Verification items for the finished model (mm, model axes). A direction names the side the tool comes from. Give positions to 0.01 mm unless a question says otherwise; leave off trailing zeros. Order: outer loops, then holes, each group sorted by start corner. A loop starts at its lowest first (then second) coordinate and runs counter-clockwise, first axis right, second up. Notation, with made-up numbers: M 65,19 L 116,19 A33 ccw 116,56 Z; hole C 72,47.5 d3. An arc over 180 degrees is marked long. Answer as a JSON object with one key per item and string values.
```python
from build123d import *

# Parameters (mm, degrees)
F0_W      = 65
F0_H      = 36
F1_DEPTH  = 23
F2_W      = 56
F2_H      = 26
F3_DEPTH  = 20
F4_R      = 2
F5_DEPTH  = 2
F6_R      = 1.25
F7_DEPTH  = 3
F8_R      = 1.25
F9_DEPTH  = 3
F10_R     = 6
F10_R_2   = 1.5
F11_DEPTH = 5
F12_W     = 24
F12_H     = 6
F13_DEPTH = 100


with BuildPart() as f1:
    # F0 (on Top) → F1 (new body)
    with BuildSketch(Plane.XY):
        Rectangle(F0_W, F0_H)
    extrude(amount=F1_DEPTH)

    # F2 (on face) → F3 (cut)
    with BuildSketch(Plane.XY.offset(23)):
        Rectangle(F2_W, F2_H)
    extrude(amount=-F3_DEPTH, mode=Mode.SUBTRACT)

    # F4 (on face) → F5 (join)
    with BuildSketch(Plane.XY.offset(3)):
        with Locations((-17, 9.5)):
            Circle(F4_R)
        with Locations((16.5, -9.5)):
            Circle(F4_R)
    extrude(amount=F5_DEPTH)

    # F6 (on face) → F7 (cut)
    with BuildSketch(Plane.XY.offset(5)):
        with Locations((-17, 9.5)):
            Circle(F6_R)
    extrude(amount=-F7_DEPTH, mode=Mode.SUBTRACT)

    # F8 (on face) → F9 (cut)
    with BuildSketch(Plane.XY.offset(5)):
        with Locations((16.5, -9.5)):
            Circle(F8_R)
    extrude(amount=-F9_DEPTH, mode=Mode.SUBTRACT)

    # F10 (on face) → F11 (join)
    with BuildSketch(Plane(origin=(0, 0, 0), x_dir=(1, 0, 0), z_dir=(0, 0, -1))):
        with Locations((-32.5, 18)):
            Circle(F10_R)
        with Locations((-34.5, 20)):
            Circle(F10_R_2, mode=Mode.SUBTRACT)
        with Locations((32.5, 18)):
            Circle(F10_R)
        with Locations((34.5, 20)):
            Circle(F10_R_2, mode=Mode.SUBTRACT)
        with Locations((32.5, -18)):
            Circle(F10_R)
        with Locations((34.5, -20)):
            Circle(F10_R_2, mode=Mode.SUBTRACT)
        with Locations((-32.5, -18)):
            Circle(F10_R)
        with Locations((-34.5, -20)):
            Circle(F10_R_2, mode=Mode.SUBTRACT)
    extrude(amount=-F11_DEPTH)

    # F12 (on face) → F13 (cut)
    with BuildSketch(Plane.YZ.offset(32.5)):
        with Locations((0, 9)):
            Rectangle(F12_W, F12_H)
    extrude(amount=-F13_DEPTH, mode=Mode.SUBTRACT)


solid = f1.part
```
Q1. Gauge pin test, flat ends, axial feed: pin 1 Ø11.5 at (y, z) = (-6.5, 16.5) entering from +X; pin 2 Ø2 at (x, z) = (-19, 11) entering from +Y; pin 3 Ø1 at (x, z) = (28, 10.5) entering from -Y. Record the tip position at first contact, or that the pin passes through.
Resolved:
{"pin 1": "stops at x = 32.5", "pin 2": "stops at y = 18", "pin 3": "stops at y = -18"}
Q2. Section check D-D on x = -1.5. Record the cut outline in (y, z), then the cut area to 3 significant figures.
Resolved:
{"outline": "M -18,0 L 18,0 L 18,23 L 13,23 L 13,3 L -13,3 L -13,23 L -18,23 Z", "area": "308 mm²"}
Q3. Section check B-B on z = 7. Record the cut outline in (x, y).
Resolved:
{"outline": "M -32.5,-18 L 32.5,-18 L 32.5,-12 L 28,-12 L 28,-13 L -28,-13 L -28,-12 L -32.5,-12 Z; M -32.5,12 L -28,12 L -28,13 L 28,13 L 28,12 L 32.5,12 L 32.5,18 L -32.5,18 Z"}
Q4. Release check for a two-part mould opening along X. For faces 5 (the face through (-33, -18, 5)), 6 (the face through (-18.474, 10.852, 3.986)), 7 (the face through (-32.5, 0, 14)) record: +X half, -X half, draft (parallel to the pull), parting line (faces both ways), or undercut.
Resolved:
{"face 5": "draft", "face 6": "undercut", "face 7": "-X half"}
Q5. Section check C-C on z = 14.5. Record the cut outline in (x, y).
Resolved:
{"outline": "M -32.5,-18 L 32.5,-18 L 32.5,18 L -32.5,18 Z; hole M -28,-13 L 28,-13 L 28,13 L -28,13 Z"}
Q6. Tool access check on faces 1 (the face through (-36.6, -22.38, 2.46)), 2 (the face through (30, 12, 9)), 3 (the face through (-17, 10, 2)), 4 (the face through (0, -18, 11)). Record the directions out of +Z, -Z, +X, -X, +Y, -Y that give a thin tool (end or side, any length) a straight path to the whole face; none if there is none.
Resolved:
{"face 1": "+Z, -Z", "face 2": "+X, -X", "face 3": "+Z", "face 4": "+Z, -Y"}
Q7. Section check A-A on y = -0.5. Record the cut outline in (x, z).
Resolved:
{"outline": "M -32.5,0 L 32.5,0 L 32.5,6 L 28,6 L 28,3 L -28,3 L -28,6 L -32.5,6 Z; M -32.5,12 L -28,12 L -28,23 L -32.5,23 Z; M 28,12 L 32.5,12 L 32.5,23 L 28,23 Z"}
Q8. Material ranges on L1, parallel to Y at x = -0.5, z = 7.5; L2, parallel to X at y = 20, z = 3.1; L3, parallel to Y at x = 34.5, z = 1.2, recorded low to high.
Resolved:
{"L1": "y = -18 to -13, 13 to 18", "L2": "x = -38.16 to -36, -33 to -26.84, 26.84 to 33, 36 to 38.16", "L3": "y = -23.66 to -21.5, -18.5 to -12.34, 12.34 to 18.5, 21.5 to 23.66"}
